Autodesk Inventor part; units mm, degrees
ref_plane "YZ Plane" through (0, 0, 0) normal (1, 0, 0) x (0, 1, 0)
ref_plane "XZ Plane" through (0, 0, 0) normal (0, 1, 0) x (-1, 0, 0)
ref_plane "XY Plane" through (0, 0, 0) normal (0, 0, 1) x (1, 0, 0)
sketch "Sketch1" plane through (0, 0, 0) normal (0, 1, 0) x (-1, 0, 0)
  circle A0 centre (0, 0) radius 20
  dimension "d0" = 40
extrude "Extrusion1" add sketch "Sketch1" along normal blind 37
sketch "Sketch2" plane through (0, 37, 0) normal (0, 1, 0) x (1, 0, 0)
  circle A0 centre (0, 0) radius 31
  dimension "d3" = 62
extrude "Extrusion2" add sketch "Sketch2" along normal blind 5
chamfer "Chamfer1" distance 2 angle 45 1 edges at (20, 0, 0)
sketch "Sketch3" plane through (0, 0, 0) normal (0, -1, 0) x (1, 0, 0)
  line L0 (13.2, 13.2) -> (-13.2, 13.2)
  line L1 (-13.2, 13.2) -> (-13.2, -13.2)
  line L2 (-13.2, -13.2) -> (13.2, -13.2)
  line L3 (13.2, -13.2) -> (13.2, 13.2)
  point P0 (0, 0)
  dimension "d9" = 26.4
  dimension "d10" = 26.4
extrude "Extrusion3" cut sketch "Sketch3" against normal blind 50
sketch "Sketch4" plane through (0, 0, 0) normal (0, -1, 0) x (1, 0, 0)
  circle A0 centre (16.2, 0) radius 2
  circle A1 centre (-16.2, 0) radius 2
  point P0 (0, 0)
  dimension "d13" = 4
  dimension "d14" = 4
extrude "Extrusion4" cut sketch "Sketch4" against normal blind 50
sketch "Sketch5" plane through (0, 42, 0) normal (0, 1, 0) x (1, 0, 0)
  line L0 (12.2376, 13.2) -> (-12.2376, 13.2)
  line L1 (10, 13.2) -> (-10, 13.2)
  line L2 (-10, 13.2) -> (-10, 18.2)
  line L3 (-10, 18.2) -> (10, 18.2)
  line L4 (10, 18.2) -> (10, 13.2)
  line L5 (-12.2376, -13.2) -> (12.2376, -13.2)
  line L6 (10, -13.2) -> (-10, -13.2)
  line L7 (-10, -13.2) -> (-10, -18.2)
  line L8 (-10, -18.2) -> (10, -18.2)
  line L9 (10, -18.2) -> (10, -13.2)
  point P0 (0, 0)
  dimension "d17" = 20
  dimension "d18" = 5
  dimension "d19" = 20
  dimension "d20" = 5
extrude "Extrusion5" add sketch "Sketch5" along normal blind 25.6
fillet "Fillet1" radius 10 4 edges at (10, 67.6, -15.7) (-10, 67.6, -15.7) (10, 67.6, 15.7) (-10, 67.6, 15.7)
sketch "Sketch6" plane through (-10, 42, 18.2) normal (0, 0, 1) x (1, 0, 0)
  circle A0 centre (10, 15.6) radius 2
  line L0 (20, 0) -> (0, 0)
  point P0 (10, -42)
  dimension "d24" = 4
  dimension "d31" = 15.6
extrude "Extrusion6" cut sketch "Sketch6" against normal blind 50
fillet "Fillet2" radius 2 7 edges at (-31, 42, 0) (10, 49.8, 18.2) (-10, 49.8, 18.2) (7.0711, 64.6711, 18.2) (-10, 49.8, -18.2) (10, 49.8, -18.2) (7.0711, 64.6711, -18.2)
chamfer "Chamfer2" distance 2 angle 45 1 edges at (-31, 37, 0)
properties part number "bigSpringMountT"
Work out the finished part from the listing and answer in its coordinate system (mm). A direction names the side the tool comes from. Round coordinates to 2 decimals unless told otherwise and drop trailing zeros.
1) Consider probe 1 along Y at (x, z) = (0, -15); probe 2 along Z at (x, y) = (-6, 53); probe 3 along Z at (x, y) = (4.5, 21). Determine where each line is inside the solid, lowest interval first.
2) Flat-ended cylindrical pins translate along their axes: P1, Ø8, axis at x = 0, y = 51, coming from the -Z side; P2, Ø3.5, axis at y = 50, z = 15, coming from the -X side; P3, Ø4, axis at y = 23.5, z = -8.5, coming from the +X side; P4, Ø6.5, axis at x = -16.2, z = 0, coming from the -Y side. Find the tip coordinate at first contact, or state that the pin passes through.
3) A cutting plane is placed at A-A on x = 1. Give the number of separate pieces and of enclosed holes in the cut face, and give its area (3 significant figures).
4) Determine the mould class of faces 1 (the face through (4.336, 19.255, 19.524)), 2 (the face through (0, 0, 15)), 3 (the face through (6.99, 64.75, 14.68)), 4 (the face through (-18.198, 20.706, 0.088)) for opening direction X: pulls with the +X half, pulls with the -X half, needs draft (parallel to the pull), parting line crosses it, or undercut.
5) Which of the six approach directions +Z, -Z, +X, -X, +Y, -Y give full straight-line access (tool end or side, diameter ignored) to faces 5 (the face through (-10, 50, 15)), 6 (the face through (9.4, 49.69, -17.63)), 7 (the face through (10, 50, -15))?
Entries:
1. probe 1: y = 0 to 55.6, 59.6 to 67.6
1. probe 2: z = -18.2 to -13.2, 13.2 to 18.2
1. probe 3: z = -19.49 to -13.2, 13.2 to 19.49
2. P1: stops at z = -18.2
2. P2: stops at x = -10
2. P3: stops at x = 18.91
2. P4: stops at y = 0
3. separate pieces: 4
3. enclosed holes: 0
3. area: 889 mm2
4. face 1: parting line crosses it
4. face 2: needs draft
4. face 3: pulls with the +X half
4. face 4: undercut
5. face 5: +Z, -Z, -X, +Y
5. face 6: -Z, +X, +Y
5. face 7: +Z, -Z, +X, +Y
